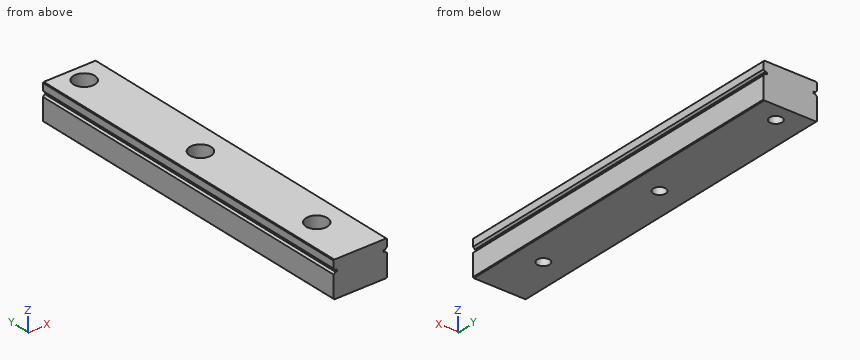
from build123d import *

# Parameters (mm, degrees)
F1_DEPTH = 100
F2_R     = 1.75
F3_DEPTH = 10.001
F2_R_2   = 3
F4_DEPTH = 4.5


with BuildPart() as f1:
    # F0 (on Front) → F1 (new body)
    with BuildSketch(Plane.XZ):
        Polygon((6.980425, 12.446069), (6.980425, 6.346069), (7.180425, 6.146069), (21.780425, 6.146069), (21.980425, 6.346069), (21.980425, 12.446069), (21.480425, 12.946069), (20.980425, 12.946069), (20.980425, 13.446069), (21.480425, 13.446069), (21.980425, 13.946069), (21.980425, 15.946069), (21.780425, 16.146069), (7.180425, 16.146069), (6.980425, 15.946069), (6.980425, 13.946069), (7.480425, 13.446069), (7.980425, 13.446069), (7.980425, 12.946069), (7.480425, 12.946069), align=None)
    extrude(amount=F1_DEPTH)

    # F2 (on face) → F3 (cut, through all)
    with BuildSketch(Plane.XY.offset(16.146069)):
        with Locations((14.480425, -85)):
            Circle(F2_R)
        with Locations((14.480425, -45)):
            Circle(F2_R)
        with Locations((14.480425, -5)):
            Circle(F2_R)
    extrude(amount=-F3_DEPTH, mode=Mode.SUBTRACT)

    # F2 (on face) → F4 (cut)
    with BuildSketch(Plane.XY.offset(16.146069)):
        with Locations((14.480425, -85)):
            Circle(F2_R_2)
        with Locations((14.480425, -85)):
            Circle(F2_R, mode=Mode.SUBTRACT)
        with Locations((14.480425, -45)):
            Circle(F2_R_2)
        with Locations((14.480425, -45)):
            Circle(F2_R, mode=Mode.SUBTRACT)
        with Locations((14.480425, -5)):
            Circle(F2_R_2)
        with Locations((14.480425, -5)):
            Circle(F2_R, mode=Mode.SUBTRACT)
    extrude(amount=-F4_DEPTH, mode=Mode.SUBTRACT)


solid = f1.part
Geometry check sheet. Reference: the model listing, model coordinates, mm. Give positions to 0.01 mm unless a question says otherwise; leave off trailing zeros. Order: outer loops, then holes, each group sorted by start corner. A loop starts at its lowest first (then second) coordinate and runs counter-clockwise, first axis right, second up. Notation, with made-up numbers: (21.5, 36.25) - (61.5, 36.25) arc R7 cw to (61.5, 45.25) - close; hole circle Ø11 at (-35, 70). An arc over 180 degrees is marked (long way). Answer as a JSON object with one key per item and string values.
(1) Material ranges on line 1 (Y direction, x = 15, z = 7.75); line 2 (Y direction, x = 13, z = 9); line 3 (X direction, y = -47, z = 12.25), recorded low to high.
Report:
{"line 1": "-100 to -86.67, -83.33 to -46.67, -43.33 to -6.67, -3.33 to 0", "line 2": "-100 to -85.93, -84.07 to -45.93, -44.07 to -5.93, -4.07 to 0", "line 3": "6.98 to 12.24, 16.72 to 21.98"}
(2) Cross-section at B-B (z = 10.75). Record the cut outline in (x, y), then the cut area to 3 significant figures.
Report:
{"outline": "(6.98, -100) - (21.98, -100) - (21.98, 0) - (6.98, 0) - close; hole circle Ø3.5 at (14.48, -85); hole circle Ø3.5 at (14.48, -45); hole circle Ø3.5 at (14.48, -5)", "area": "1,470 mm^2"}
(3) Cross-section at C-C (x = 15.25). Record the cut outline in (y, z).
Report:
{"outline": "(-100, 6.15) - (-86.57, 6.15) - (-86.57, 11.65) - (-87.9, 11.65) - (-87.9, 16.15) - (-100, 16.15) - close; (-83.43, 6.15) - (-46.57, 6.15) - (-46.57, 11.65) - (-47.9, 11.65) - (-47.9, 16.15) - (-82.1, 16.15) - (-82.1, 11.65) - (-83.43, 11.65) - close; (-43.43, 6.15) - (-6.57, 6.15) - (-6.57, 11.65) - (-7.9, 11.65) - (-7.9, 16.15) - (-42.1, 16.15) - (-42.1, 11.65) - (-43.43, 11.65) - close; (-3.43, 6.15) - (0, 6.15) - (0, 16.15) - (-2.1, 16.15) - (-2.1, 11.65) - (-3.43, 11.65) - close"}
(4) Depth check by flat-ended pin: pin 1 Ø3 at (x, z) = (12, 11.5) entering from +Y; pin 2 Ø3 at (x, y) = (14, -45.5) entering from +Z. Enter the tip coordinate at first touch or a pass-through.
Report:
{"pin 1": "y = 0", "pin 2": "z = 11.65"}
(5) Cross-section at A-A (y = -85). Record the cut outline in (x, z), then the cut area to 3 significant figures.
Report:
{"outline": "(6.98, 6.35) - (7.18, 6.15) - (12.73, 6.15) - (12.73, 11.65) - (11.48, 11.65) - (11.48, 16.15) - (7.18, 16.15) - (6.98, 15.95) - (6.98, 13.95) - (7.48, 13.45) - (7.98, 13.45) - (7.98, 12.95) - (7.48, 12.95) - (6.98, 12.45) - close; (16.23, 6.15) - (21.78, 6.15) - (21.98, 6.35) - (21.98, 12.45) - (21.48, 12.95) - (20.98, 12.95) - (20.98, 13.45) - (21.48, 13.45) - (21.98, 13.95) - (21.98, 15.95) - (21.78, 16.15) - (17.48, 16.15) - (17.48, 11.65) - (16.23, 11.65) - close", "area": "102 mm^2"}
